Source: CAD feature listing. Evaluate the final solid. Frame: model axes, mm. Face numbers are marked on the shaded views. A direction names the side the tool comes from. Coordinates: 2 decimals unless noted, no trailing zeros. Loops run counter-clockwise (first coordinate to the right, second up) from the corner with the lowest first, then second, coordinate; pieces in that order, holes last. Notation, with made-up numbers: M 9,-40 L 65,-40 A24 cw 65,-1 Z; hole C -2.5,31 d8. An arc over 180 degrees is marked long. One line per question, with ' | ' between items. Start each with the question number.
1. Section query D-D, the plane z = -64. Output: boundary loops of the cut face in (x, y).
2. Section query A-A, the plane x = -13. Output: boundary loops of the cut face in (y, z), and give its area (3 significant figures).
3. Ray query, probe 1 along Z at (x, y) = (0, -11.5); probe 2 along Z at (x, y) = (27, -4.75); probe 3 along Y at (x, z) = (13, 3.05). Return the intervals inside material, ascending.
4. Access query for the marked faces 5, 6 and 7. Directions: +Z, -Z, +X, -X, +Y, -Y. A direction counts if a zero-diameter tool reaches every point of the face in a straight line with its end or side. Return the directions, or none.
5. Section query B-B, the plane x = 11.5. Output: boundary loops of the cut face in (y, z), and give its area (3 significant figures).
6. Pin query (flat end, axial travel): P1, Ø8, axis at y = -10, z = -103.5, coming from the +X side; P2, Ø1.6, axis at x = -27, y = 0, coming from the -Z side; P3, Ø0.5, axis at y = -8.5, z = -82, coming from the -X side. Return the tip coordinate at first contact, or that it passes through.
7. Section query C-C, the plane y = -3. State how many separate pieces and enclosed holes the cut face has, and give its area (3 significant figures).
8. Mould query, pull axis Z, two halves, no side actions, for the marked faces 1, 2, 3 and 4. Classes: pulls with the +Z half, pulls with the -Z half, needs draft (parallel to the pull), parting line crosses it, or undercut.
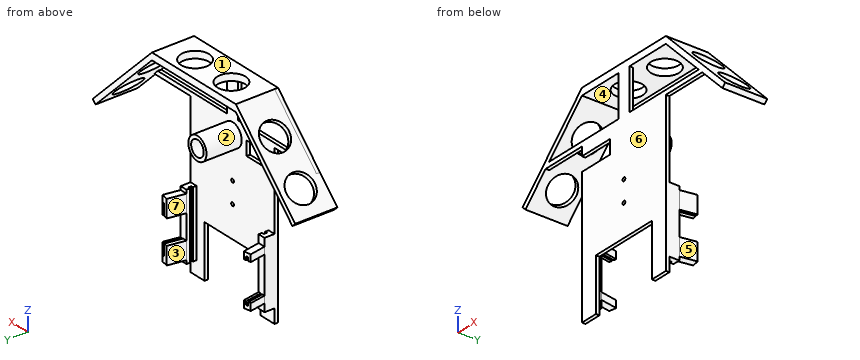
```python
from build123d import *

# Parameters (mm, degrees)
SKETCH1_W           = 60
SKETCH1_H           = 22
SKETCH1_R           = 8
BOSS_EXTRUDE1_DEPTH = 4
BOSS_EXTRUDE2_DEPTH = 2
BOSS_EXTRUDE3_START = -70
BOSS_EXTRUDE3_DEPTH = 38
BOSS_EXTRUDE5_DEPTH = 10
BOSS_EXTRUDE6_DEPTH = 10
SKETCH10_R          = 1
CUT_EXTRUDE1_DEPTH  = 4
SKETCH12_W          = 24
SKETCH12_H          = 60
SKETCH12_R          = 8
BOSS_EXTRUDE7_DEPTH = 2.83
SKETCH13_R          = 6.5
SKETCH13_R_2        = 4.5
BOSS_EXTRUDE8_DEPTH = 20


with BuildPart() as part:
    # Sketch1 → Boss-Extrude1 (new body)
    with BuildSketch(Plane.XY):
        Rectangle(SKETCH1_W, SKETCH1_H)
        with Locations((-13, 0)):
            Circle(SKETCH1_R, mode=Mode.SUBTRACT)
        with Locations((13, 0)):
            Circle(SKETCH1_R, mode=Mode.SUBTRACT)
    extrude(amount=BOSS_EXTRUDE1_DEPTH)

    # Sketch2 → Boss-Extrude2 (add)
    with BuildSketch(Plane(origin=(0, -11, 0), x_dir=(-1, 0, 0), z_dir=(0, -1, 0))):
        Polygon((-30, 116), (-20, 116), (-20, 86), (20, 86), (20, 116), (30, 116), (30, 39), (10, 39), (10, 31), (30, 31), (30, 26), (60, 26), (30.002383175, -4), (30, -4), (-30, -4), (-60, 26), (-30, 26), align=None)
        Polygon((-53.5, 23.5), (-30, 0), (-4, 0), (-4, 23.5), align=None, mode=Mode.SUBTRACT)
        Polygon((53.49813318, 23.5), (30, 0), (4, 0), (4, 23.5), align=None, mode=Mode.SUBTRACT)
    extrude(amount=BOSS_EXTRUDE2_DEPTH)

    # Sketch4 → Boss-Extrude3 (add)
    with BuildSketch(Plane.XY.offset(BOSS_EXTRUDE3_START)):
        Polygon((-25.8, -11), (-25.8, -9), (-27, -9), (-27, -7.3), (-25.8, -7.3), (-25.8, -5.3), (-30, -5.3), (-30, -11), align=None)
        Polygon((30, -5.3), (30, -11), (25.8, -11), (25.8, -9), (27, -9), (27, -7.3), (25.8, -7.3), (25.8, -5.3), align=None)
    extrude(amount=-BOSS_EXTRUDE3_DEPTH)

    # Sketch7 → Boss-Extrude5 (add)
    with BuildSketch(Plane(origin=(0.128388188, -0.728125596, 0), x_dir=(0, 0, 1), z_dir=(-0.17364817766693402, 0.9848077530122075, 0))):
        Polygon((-74.5, -26.328375369), (-74.5, -30.464567932), (-78.5, -30.464567932), (-78.5, -28.964567932), (-76.5, -28.964567932), (-76.5, -27.764567932), (-78.5, -27.764567932), (-78.5, -26.328375369), align=None)
        Polygon((-101.5, -27.764567932), (-99.5, -27.764567932), (-99.5, -26.328375369), (-103.5, -26.328375369), (-103.5, -30.464567932), (-99.5, -30.464567932), (-99.5, -28.964567932), (-101.5, -28.964567932), align=None)
    extrude(amount=BOSS_EXTRUDE5_DEPTH)

    # Sketch8 → Boss-Extrude6 (add)
    with BuildSketch(Plane(origin=(-0.128388188, -0.728125596, 0), x_dir=(0, 0, 1), z_dir=(0.17364817766692736, 0.9848077530122086, 0))):
        Polygon((-82, 26.328375369), (-82, 28.714567932), (-75.5, 28.714567932), (-75.5, 29.764567932), (-82, 29.764567932), (-82, 30.464567932), (-72, 30.464567932), (-72, 26.328375369), align=None)
        Polygon((-96, 29.764567932), (-96, 30.464567932), (-106, 30.464567932), (-106, 26.328375369), (-96, 26.328375369), (-96, 28.714567932), (-102.5, 28.714567932), (-102.5, 29.764567932), align=None)
    extrude(amount=BOSS_EXTRUDE6_DEPTH)

    # Sketch10 → Cut-Extrude1 (cut)
    with BuildSketch(Plane.XZ.offset(13)):
        with Locations((0, -56)):
            Circle(SKETCH10_R)
        with Locations((0, -68)):
            Circle(SKETCH10_R)
    extrude(amount=-CUT_EXTRUDE1_DEPTH, mode=Mode.SUBTRACT)

    # Sketch12 → Boss-Extrude7 (add)
    with BuildSketch(Plane(origin=(17, 0, 17), x_dir=(0, 1, 0), z_dir=(0.7071067811865561, 0, 0.7071067811865389))):
        with Locations((-1, -48.384776311)):
            Rectangle(SKETCH12_W, SKETCH12_H)
        with Locations(Location((0, -38.384776311, 0), (0, 0, 270))):
            Circle(SKETCH12_R, mode=Mode.SUBTRACT)
        with Locations(Location((0, -64.384776311, 0), (0, 0, 270))):
            Circle(SKETCH12_R, mode=Mode.SUBTRACT)
    boss_extrude7 = extrude(amount=-BOSS_EXTRUDE7_DEPTH)

    # Mirror2: Boss-Extrude7 across plane
    add(boss_extrude7.mirror(Plane(origin=(0, 0, 0), x_dir=(0, 0, 1), z_dir=(1, 0, 0))))

    # Sketch13 → Boss-Extrude8 (add)
    with BuildSketch(Plane(origin=(0, -11, 0), x_dir=(1, 0, 0), z_dir=(0, 1, 0))):
        with Locations(Location((0, 32.5, 0), (0, 0, 90))):
            Circle(SKETCH13_R)
        with Locations(Location((0, 32.5, 0), (0, 0, 270))):
            Circle(SKETCH13_R_2, mode=Mode.SUBTRACT)
    extrude(amount=BOSS_EXTRUDE8_DEPTH)


solid = part.part
```
Taken from the geometry:
1) outline: M -30,-13 L 30,-13 L 30,-11 L -30,-11 Z
2) outline: M -13,-86 L -11,-86 L -11,-39 L -13,-39 Z; M -13,-31 L -11,-31 L -11,-23.5 L -13,-23.5 Z; M -13,0 L -8,0 L -8,4 L -13,4 Z; M 8,0 L 11,0 L 11,4 L 8,4 Z | area: 141 mm^2
3) probe 1: -86 to -69, -67 to -57, -55 to 4 | probe 2: -106 to -96, -82 to -72, 0 to 4 | probe 3: -13 to -8, 8 to 11
4) face 5: -Z, +X, -Y | face 6: +Z, -Z, +X, -X, -Y | face 7: -Z, +Y
5) outline: M -13,-86 L -11,-86 L -11,-23.5 L -13,-23.5 Z; M -13,0 L -7.86,0 L -7.86,4 L -13,4 Z; M 7.86,0 L 11,0 L 11,4 L 7.86,4 Z | area: 158 mm^2
6) P1: x = 30 | P2: z = -103.5 | P3: x = -30
7) separate pieces: 12 | enclosed holes: 1 | area: 453 mm^2
8) face 1: pulls with the +Z half | face 2: undercut | face 3: needs draft | face 4: undercut
